Model file for the job. Use its own axes, mm. A direction names the side the tool comes from. Coordinates: 2 decimals unless noted, no trailing zeros. Order: outer loops, then holes, each group sorted by start corner. A loop starts at its lowest first (then second) coordinate and runs counter-clockwise, first axis right, second up. Notation, with made-up numbers: (-19, 58.5) -> (10, 58.5) arc R14 cw to (10, 84.5) -> close; hole circle Ø9 at (84, -3.75). An arc over 180 degrees is marked (long way). Return JSON: item names as keys, results as strings. Group by question number.
1) Cut at A-A (y = 3.5). Write the cut outline in (x, z) (1 decimal), and give its area (3 significant figures).
2) Probe line 1 (Y direction, x = 0, z = 9.5) (3 decimals); line 2 (Y direction, x = 7, z = 9.25); line 3 (X direction, y = 5.5, z = 0.5). List the from-to ranges inside material, lowest first.
3) Pull direction X, two halves, no side cores. Call faces 4 (the cylindrical face through (-7.559, -5.796, 6.261)), 5 (the cylindrical face through (18.17, 5.72, 2.37)), 6 (the flat face through (-9, 13, 3.175)): +X half, -X half, draft (parallel to the pull), parting line (faces both ways), or undercut.
4) Cut at C-C (z = 9). Write the cut outline in (x, y) (3 decimals), and give its area (3 significant figures).
5) Cut at D-D (x = -11). Write the cut outline in (y, z) (1 decimal), and give its area (3 significant figures).
6) Which spindle directions (+Z, -Z, +X, -X, +Y, -Y) get a long thin tool onto all of the face, cutting with end or side? Do faces 1 (the flat face through (7, 7, 12.7)), 2 (the cylindrical face through (12.4, -2.75, 0.78)), 3 (the cylindrical face through (-15.19, -1.99, 7.87)). Say none if no direction does.
7) Flat gauge pins, fed straight in: pin 1 (1 mm diameter, centred on x = 4, z = 11, fed in from +Y); pin 2 (8 mm diameter, centred on x = -6, y = -3, fed in from -Z); pin 3 (4 mm diameter, centred on x = 11, z = 4, fed in from +Y); pin 4 (1 mm diameter, centred on x = 3, z = 7.5, fed in from +Y). Where does each tip first touch, or does it go through?
from build123d import *

# Parameters (mm, degrees)
SKETCH1_R           = 19.05
SKETCH1_R_2         = 9.525
BOSS_EXTRUDE1_DEPTH = 12.7
SKETCH2_W           = 9.525
SKETCH2_H           = 3.729002221
SKETCH2_W_2         = 1.5875
SKETCH2_H_2         = 6.35


with BuildPart() as part:
    # Sketch1 → Boss-Extrude1 (new body)
    with BuildSketch(Plane.XY):
        Circle(SKETCH1_R)
        Circle(SKETCH1_R_2, mode=Mode.SUBTRACT)
    extrude(amount=BOSS_EXTRUDE1_DEPTH)

    # Sketch2 → Cut-Revolve1 (revolve, cut)
    with BuildSketch(Plane(origin=(0, 0, 0), x_dir=(0, 0, -1), z_dir=(1, 0, 0))):
        with Locations((-7.9375, 17.185498889)):
            Rectangle(SKETCH2_W, SKETCH2_H)
        with Locations((-0.79375, 15.875)):
            Rectangle(SKETCH2_W_2, SKETCH2_H_2)
    revolve(axis=Axis((0, 0, 0), (0, 0, 1)), mode=Mode.SUBTRACT)


solid = part.part
Answers below:
{
 "1": {"outline": "(-18.7, 1.6) -> (-12.2, 1.6) -> (-12.2, 0) -> (-8.9, 0) -> (-8.9, 12.7) -> (-14.9, 12.7) -> (-14.9, 3.2) -> (-18.7, 3.2) -> close; (8.9, 0) -> (12.2, 0) -> (12.2, 1.6) -> (18.7, 1.6) -> (18.7, 3.2) -> (14.9, 3.2) -> (14.9, 12.7) -> (8.9, 12.7) -> close", "area": "157 mm^2"},
 "2": {"line 1": "y = -15.321 to -9.525, 9.525 to 15.321", "line 2": "y = -13.63 to -6.46, 6.46 to 13.63", "line 3": "x = -11.45 to -7.78, 7.78 to 11.45"},
 "3": {"face 4": "undercut", "face 5": "parting line", "face 6": "draft"},
 "4": {"outline": "circle Ø30.642 at (0, 0); hole circle Ø19.05 at (0, 0)", "area": "452 mm^2"},
 "5": {"outline": "(-15.6, 1.6) -> (-6.3, 1.6) -> (-6.3, 0) -> (6.3, 0) -> (6.3, 1.6) -> (15.6, 1.6) -> (15.6, 3.2) -> (10.7, 3.2) -> (10.7, 12.7) -> (-10.7, 12.7) -> (-10.7, 3.2) -> (-15.6, 3.2) -> close", "area": "273 mm^2"},
 "6": {"face 1": "+Z, +X, -X, +Y, -Y", "face 2": "-Z", "face 3": "+Z"},
 "7": {"pin 1": "stops at y = 14.92", "pin 2": "stops at z = 0", "pin 3": "stops at y = 16.69", "pin 4": "stops at y = 15.12"}
}
